from build123d import *

# Parameters (mm, degrees)
F0_W     = 150
F0_H     = 100
F1_DEPTH = 30
F2_W     = 140
F2_H     = 90
F3_DEPTH = 25
F4_SIZE  = 2


with BuildPart() as f1:
    # F0 (on Top) → F1 (new body)
    with BuildSketch(Plane.XY):
        Rectangle(F0_W, F0_H)
    extrude(amount=F1_DEPTH)

    # F2 (on face) → F3 (cut)
    with BuildSketch(Plane.XY.offset(30)):
        Rectangle(F2_W, F2_H)
    extrude(amount=-F3_DEPTH, mode=Mode.SUBTRACT)

    # F4
    f4_edges = [f1.edges().sort_by_distance(p)[0] for p in [
        (-70, 0, 5),
        (0, -45, 5),
        (70, 0, 5),
        (0, 45, 5),
        (-70, 45, 17.5),
        (70, 45, 17.5),
        (70, -45, 17.5),
        (-70, -45, 17.5),
    ]]
    chamfer(f4_edges, length=F4_SIZE)


solid = f1.part
Geometry check sheet. Reference: the model listing, model coordinates, mm. A direction names the side the tool comes from. Give positions to 0.01 mm unless a question says otherwise; leave off trailing zeros. Order: outer loops, then holes, each group sorted by start corner. A loop starts at its lowest first (then second) coordinate and runs counter-clockwise, first axis right, second up. Notation, with made-up numbers: M 70.25,36.5 L 75.25,36.5 A24 cw 75.25,58.5 Z; hole C 50,-17 d7. An arc over 180 degrees is marked long. Use a Markdown table: item, result.
Item 1: Material ranges on line 1 along Y through (x, z) = (-43.5, 8.5); line 2 along X through (y, z) = (-19.5, 27); line 3 along Z through (x, y) = (-30.5, -32.5), recorded low to high.
Answers follow:
| item | result |
|---|---|
| line 1 | y = -50 to -45, 45 to 50 |
| line 2 | x = -75 to -70, 70 to 75 |
| line 3 | z = 0 to 5 |
Item 2: Tool access check on faces 4 (the flat face through (-70, -1, 19)), 5 (the flat face through (-75, -1, 15)). Record the directions out of +Z, -Z, +X, -X, +Y, -Y that give a thin tool (end or side, any length) a straight path to the whole face; none if there is none.
Answers follow:
| item | result |
|---|---|
| face 4 | +Z |
| face 5 | +Z, -Z, -X, +Y, -Y |
Item 3: Section check B-B (z = 18). Record the cut outline in (x, y).
Answers follow:
| item | result |
|---|---|
| outline | M -75,-50 L 75,-50 L 75,50 L -75,50 Z; hole M -70,-43 L -68,-45 L 68,-45 L 70,-43 L 70,43 L 68,45 L -68,45 L -70,43 Z |
Item 4: Draft check along Y on faces 1 (the flat face through (-6, -48, 30)), 2 (the flat face through (70, -1, 19)), 3 (the flat face through (-1, -50, 15)). Enter one of: +Y half, -Y half, draft (parallel to the pull), parting line (faces both ways), or undercut.
Answers follow:
| item | result |
|---|---|
| face 1 | draft |
| face 2 | undercut |
| face 3 | -Y half |
Item 5: Section check A-A (y = 6.5). Record the cut outline in (x, z), and give its area (3 significant figures).
Answers follow:
| item | result |
|---|---|
| outline | M -75,0 L 75,0 L 75,30 L 70,30 L 70,7 L 68,5 L -68,5 L -70,7 L -70,30 L -75,30 Z |
| area | 1,000 mm2 |
Item 6: Depth check by flat-ended pin: P1, Ø10, axis at x = -59, y = 10.5, coming from the +Z side. Enter the tip coordinate at first touch or a pass-through.
Answers follow:
| item | result |
|---|---|
| P1 | stops at z = 5 |
Item 7: Section check C-C (x = -7). Record the cut outline in (y, z), and give its area (3 significant figures).
Answers follow:
| item | result |
|---|---|
| outline | M -50,0 L 50,0 L 50,30 L 45,30 L 45,7 L 43,5 L -43,5 L -45,7 L -45,30 L -50,30 Z |
| area | 754 mm2 |
